from build123d import *
from OCP.BRepFilletAPI import BRepFilletAPI_MakeChamfer

# Parameters (mm, degrees)
SKETCH1_W                                  = 42.3
SKETCH1_H                                  = 5.8
SKETCH1_W_2                                = 41.5
SKETCH1_H_2                                = 5
CORE_POCKET_DEPTH                          = 27
SKETCH2_W                                  = 41
SKETCH2_H                                  = 4.5
BOSS_EXTRUDE2_DEPTH                        = 4.1
CHAMFER2_SIZE                              = 1.1
CHAMFER2_SIZE_2                            = 0.635085296
CHAMFER3_SIZE                              = 1.417820455
CHAMFER3_SIZE_2                            = 0.25
SIDE_SUPPORT_DEPTH                         = 2.9
SIDE_SUPPORT_FILLET_R                      = 0.65
SIDE_SUPPORT_FILLET_OF_SIDE_SUPPORT_MIRR_R = 0.65
BOSS_EXTRUDE3_START                        = 4.1
SKETCH5_W                                  = 3
SKETCH5_H                                  = 0.25
BOSS_EXTRUDE3_DEPTH                        = 45.8
FILLET1_R                                  = 0.25


# Read off the part's stored shape, not the designer's step: Mirror1
# Some blends are built 0.0001 mm under size
with BuildPart() as part:
    # Sketch1 → Core-Pocket (new, symmetric)
    with BuildSketch(Plane.XY):
        Rectangle(SKETCH1_W, SKETCH1_H)
        Rectangle(SKETCH1_W_2, SKETCH1_H_2, mode=Mode.SUBTRACT)
    extrude(amount=CORE_POCKET_DEPTH, both=True)

    # Sketch2 → Boss-Extrude2 (add)
    with BuildSketch(Plane.XY.offset(27)):
        with BuildLine():
            Line((-22, -4), (22, -4))
            ThreePointArc((22, -4), (23.414213562, -3.414213562), (24, -2))
            Line((24, -2), (24, 2))
            ThreePointArc((24, 2), (23.414213562, 3.414213562), (22, 4))
            Line((22, 4), (-22, 4))
            ThreePointArc((-22, 4), (-23.414213562, 3.414213562), (-24, 2))
            Line((-24, 2), (-24, -2))
            ThreePointArc((-24, -2), (-23.414213562, -3.414213562), (-22, -4))
        make_face()
        Rectangle(SKETCH2_W, SKETCH2_H, mode=Mode.SUBTRACT)
    extrude(amount=-BOSS_EXTRUDE2_DEPTH)

    # Chamfer2
    chamfer2_edges_1 = [part.edges().sort_by_distance(p)[0] for p in [
        (23.414213562, 3.414213562, 22.9),
    ]]
    chamfer2_side_1 = [part.faces().sort_by_distance(p)[0] for p in [
        (23.4052321, 3.4052321, 22.9),
    ]]
    chamfer2_edges_2 = [part.edges().sort_by_distance(p)[0] for p in [
        (24, 0, 22.9),
    ]]
    chamfer2_side_2 = [part.faces().sort_by_distance(p)[0] for p in [
        (23.987298294, 0, 22.9),
    ]]
    chamfer2_edges_3 = [part.edges().sort_by_distance(p)[0] for p in [
        (23.414213562, -3.414213562, 22.9),
    ]]
    chamfer2_side_3 = [part.faces().sort_by_distance(p)[0] for p in [
        (23.4052321, -3.4052321, 22.9),
    ]]
    chamfer2_edges_4 = [part.edges().sort_by_distance(p)[0] for p in [
        (0, -4, 22.9),
    ]]
    chamfer2_side_4 = [part.faces().sort_by_distance(p)[0] for p in [
        (0, -3.987298294, 22.9),
    ]]
    chamfer2_edges_5 = [part.edges().sort_by_distance(p)[0] for p in [
        (-23.414213562, -3.414213562, 22.9),
    ]]
    chamfer2_side_5 = [part.faces().sort_by_distance(p)[0] for p in [
        (-23.4052321, -3.4052321, 22.9),
    ]]
    chamfer2_edges_6 = [part.edges().sort_by_distance(p)[0] for p in [
        (-24, 0, 22.9),
    ]]
    chamfer2_side_6 = [part.faces().sort_by_distance(p)[0] for p in [
        (-23.987298294, 0, 22.9),
    ]]
    chamfer2_edges_7 = [part.edges().sort_by_distance(p)[0] for p in [
        (-23.414213562, 3.414213562, 22.9),
    ]]
    chamfer2_side_7 = [part.faces().sort_by_distance(p)[0] for p in [
        (-23.4052321, 3.4052321, 22.9),
    ]]
    chamfer2_edges_8 = [part.edges().sort_by_distance(p)[0] for p in [
        (0, 4, 22.9),
    ]]
    chamfer2_side_8 = [part.faces().sort_by_distance(p)[0] for p in [
        (0, 3.987298294, 22.9),
    ]]
    chamfer2 = BRepFilletAPI_MakeChamfer(part.part.solid().wrapped)
    for e in chamfer2_edges_1:
        chamfer2.Add(CHAMFER2_SIZE - 0.0001, CHAMFER2_SIZE_2 - 0.0001, e.wrapped, chamfer2_side_1[0].wrapped)
    for e in chamfer2_edges_2:
        chamfer2.Add(CHAMFER2_SIZE - 0.0001, CHAMFER2_SIZE_2 - 0.0001, e.wrapped, chamfer2_side_2[0].wrapped)
    for e in chamfer2_edges_3:
        chamfer2.Add(CHAMFER2_SIZE - 0.0001, CHAMFER2_SIZE_2 - 0.0001, e.wrapped, chamfer2_side_3[0].wrapped)
    for e in chamfer2_edges_4:
        chamfer2.Add(CHAMFER2_SIZE - 0.0001, CHAMFER2_SIZE_2 - 0.0001, e.wrapped, chamfer2_side_4[0].wrapped)
    for e in chamfer2_edges_5:
        chamfer2.Add(CHAMFER2_SIZE - 0.0001, CHAMFER2_SIZE_2 - 0.0001, e.wrapped, chamfer2_side_5[0].wrapped)
    for e in chamfer2_edges_6:
        chamfer2.Add(CHAMFER2_SIZE - 0.0001, CHAMFER2_SIZE_2 - 0.0001, e.wrapped, chamfer2_side_6[0].wrapped)
    for e in chamfer2_edges_7:
        chamfer2.Add(CHAMFER2_SIZE - 0.0001, CHAMFER2_SIZE_2 - 0.0001, e.wrapped, chamfer2_side_7[0].wrapped)
    for e in chamfer2_edges_8:
        chamfer2.Add(CHAMFER2_SIZE - 0.0001, CHAMFER2_SIZE_2 - 0.0001, e.wrapped, chamfer2_side_8[0].wrapped)
    add(Compound.cast(chamfer2.Shape()), mode=Mode.REPLACE)  # a hair under: the kernel refuses the full size

    # Chamfer3
    # the kernel refuses this chamfer: 1.417820455, 0.25 mm, written as the material it adds along each edge
    with BuildSketch(Plane(origin=(-20.75, 2.5, 22.9), x_dir=(0, 0.006682531656101647, -0.9999776716360547), z_dir=(1, 0, 0)), Plane(origin=(20.75, -2.5, 22.9), x_dir=(0, -0.006682531656101647, -0.9999776716360547), z_dir=(-1, 0, 0))) as chamfer3_piece_1:
        Polygon((CHAMFER3_SIZE * 0.999977671569, -CHAMFER3_SIZE * 0.00668253165565), (-CHAMFER3_SIZE_2 * 0.0066825316561, -CHAMFER3_SIZE_2 * 0.999977671636), (0, 0), align=None)
    extrude(amount=41.5)
    with BuildSketch(Plane(origin=(-20.75, -2.5, 22.9), x_dir=(-0.006682531656101949, 0, -0.9999776716360547), z_dir=(0, 1, 0)), Plane(origin=(20.75, 2.5, 22.9), x_dir=(0.006682531656101949, 0, -0.9999776716360547), z_dir=(0, -1, 0))) as chamfer3_piece_2:
        Polygon((CHAMFER3_SIZE * 0.999977671569, -CHAMFER3_SIZE * 0.00668253165565), (-CHAMFER3_SIZE_2 * 0.0066825316561, -CHAMFER3_SIZE_2 * 0.999977671636), (0, 0), align=None)
    extrude(amount=5)

    # Mirror1: part across plane


with BuildPart() as part_1:
    add(part.part)
    add(part.part.mirror(Plane.XY))

    # Sketch4 → Side support (add, symmetric)
    with BuildSketch(Plane(origin=(0, 0, 0), x_dir=(1, 0, 0), z_dir=(0, 1, 0))):
        with BuildLine():
            Line((21.15, -22.9), (22.9, -22.9))
            ThreePointArc((22.9, -22.9), (25.15, 0), (22.9, 22.9))
            Line((22.9, 22.9), (21.15, 22.9))
            ThreePointArc((21.15, 22.9), (22.65, 0), (21.15, -22.9))
        make_face()
    side_support = extrude(amount=SIDE_SUPPORT_DEPTH, both=True)

    # side support fillet
    side_support_fillet_edges = [part_1.edges().sort_by_distance(p)[0] for p in [
        (25.15, 2.9, 0),
        (25.15, -2.9, 0),
    ]]
    fillet(side_support_fillet_edges, radius=SIDE_SUPPORT_FILLET_R)

    # Side support mirror: Side support across plane
    add(side_support.mirror(Plane(origin=(0, 0, 0), x_dir=(0, 0, 1), z_dir=(1, 0, 0))))

    # side support fillet of Side support mirr
    side_support_fillet_of_side_support_mirr_edges = [part_1.edges().sort_by_distance(p)[0] for p in [
        (-25.15, 2.9, 0),
        (-25.15, -2.9, 0),
    ]]
    fillet(side_support_fillet_of_side_support_mirr_edges, radius=SIDE_SUPPORT_FILLET_OF_SIDE_SUPPORT_MIRR_R)

    # Sketch5 → Boss-Extrude3 (add)
    with BuildSketch(Plane.XY.offset(-27).offset(BOSS_EXTRUDE3_START)):
        with Locations((-12.5, -2.375)):
            Rectangle(SKETCH5_W, SKETCH5_H)
        with Locations((12.5, -2.375)):
            Rectangle(SKETCH5_W, SKETCH5_H)
        with Locations((12.5, 2.375)):
            Rectangle(SKETCH5_W, SKETCH5_H)
        with Locations((-12.5, 2.375)):
            Rectangle(SKETCH5_W, SKETCH5_H)
    extrude(amount=BOSS_EXTRUDE3_DEPTH)

    # Fillet1
    fillet1_edges = [part_1.edges().sort_by_distance(p)[0] for p in [
        (14, -2.25, 0),
        (11, -2.25, 0),
        (-14, -2.25, 0),
        (-11, -2.25, 0),
    ]]
    fillet(fillet1_edges, radius=FILLET1_R - 0.0001)  # a hair under: the kernel refuses the full size


solid = part_1.part
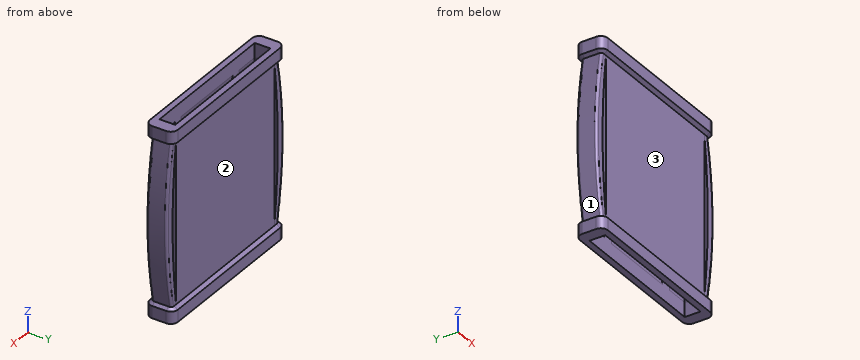
Geometry: final body of the model. Coordinates: model frame, mm. Face numbers are marked on the shaded views. A direction names the side the tool comes from. Give positions to 0.01 mm unless a question says otherwise; leave off trailing zeros. Put each result on its own line as item: value.
1) Material intervals for L1, parallel to Y at x = -16, z = -4; L2, parallel to X at y = 0.5, z = 1.5; L3, parallel to X at y = -1, z = 9, sorted ascending. Write a range as from..to.
Computed values:
L1: y = -2.9..-2.5, 2.5..2.9
L2: x = -25.14..-22.64, -21.15..-20.75, 20.75..21.15, 22.64..25.14
L3: x = -24.81..-22.42, -21.15..-20.75, 20.75..21.15, 22.42..24.81
2) Cut plane A-A, the plane y = -0.5. Give the number of separate pieces and of enclosed holes in the cut face, plus the area to 3 significant figures.
Computed values:
separate pieces: 2
enclosed holes: 2
area: 300 mm^2
3) First-contact query: P1, Ø4, axis at y = 0.5, z = -25.5, coming from the +X side; P2, Ø2, axis at y = 0, z = 3.5, coming from the -X side; P3, Ø2.5, axis at y = -0.5, z = 3.5, coming from the +X side. Flat tips, straight axial feed; report the tip coordinate or a pass-through.
Computed values:
P1: stops at x = 24
P2: stops at x = -25.12
P3: stops at x = 25.13
4) Reachability of the marked faces 1, 2 and 3 from +Z, -Z, +X, -X, +Y, -Y: full face, straight path, thin tool, end or side. Return the list, or none.
Computed values:
face 1: -X, +Y, -Y
face 2: +X, -X, +Y
face 3: +X, -X, -Y
